```python
from build123d import *

# Parameters (mm, degrees)
SK_MAIN_EXTRUSION_R  = 3.4
MAIN_EXTRUSION_DEPTH = 25


with BuildPart() as part:
    # Sk Main Extrusion → Main Extrusion (new body)
    with BuildSketch(Plane.XY):
        with BuildLine():
            Line((-16.671180212, -4.190076845), (-19.506515107, -5.222054351))
            ThreePointArc((-19.506515107, -5.222054351), (-19.864364033, -5.496641489), (-20, -5.926823816))
            Line((-20, -5.926823816), (-20, -18.5))
            ThreePointArc((-20, -18.5), (-19.560660172, -19.560660172), (-18.5, -20))
            Line((-18.5, -20), (37.5, -20))
            ThreePointArc((37.5, -20), (38.560660172, -19.560660172), (39, -18.5))
            Line((39, -18.5), (39, -16.5))
            ThreePointArc((39, -16.5), (38.560660172, -15.439339828), (37.5, -15))
            Line((37.5, -15), (31.319331136, -15))
            ThreePointArc((31.319331136, -15), (31.252521542, -15.009092387), (31.190571617, -15.035708175))
            Line((31.190571617, -15.035708175), (30.378759519, -15.523494095))
            ThreePointArc((30.378759519, -15.523494095), (30.25, -15.55920227), (30.121240481, -15.523494095))
            Line((30.121240481, -15.523494095), (29.309428383, -15.035708175))
            ThreePointArc((29.309428383, -15.035708175), (29.247478458, -15.009092387), (29.180668864, -15))
            Line((29.180668864, -15), (21, -15))
            ThreePointArc((21, -15), (20.292893219, -14.707106781), (20, -14))
            Line((20, -14), (20, -5.926823816))
            ThreePointArc((20, -5.926823816), (19.864364033, -5.496641489), (19.506515107, -5.222054351))
            Line((19.506515107, -5.222054351), (16.671180212, -4.190076845))
            ThreePointArc((16.671180212, -4.190076845), (16.563886241, -4.175951325), (16.460675177, -4.208493649))
            Line((16.460675177, -4.208493649), (15.111296024, -4.987558066))
            Line((15.111296024, -4.987558066), (14.845251581, -5.718509166))
            Line((14.845251581, -5.718509166), (15.81984631, -8.396186179))
            ThreePointArc((15.81984631, -8.396186179), (15.786489799, -8.811074612), (15.450654467, -9.056960151))
            ThreePointArc((15.450654467, -9.056960151), (12.665882372, -8.933433013), (10.272684887, -7.504160339))
            Line((10.272684887, -7.504160339), (9.309262274, -6.540737726))
            ThreePointArc((9.309262274, -6.540737726), (6.6, 0), (9.309262274, 6.540737726))
            Line((9.309262274, 6.540737726), (10.272684887, 7.504160339))
            ThreePointArc((10.272684887, 7.504160339), (12.665882372, 8.933433013), (15.450654467, 9.056960151))
            ThreePointArc((15.450654467, 9.056960151), (15.786489799, 8.811074612), (15.81984631, 8.396186179))
            Line((15.81984631, 8.396186179), (14.845251581, 5.718509166))
            Line((14.845251581, 5.718509166), (15.111296024, 4.987558066))
            Line((15.111296024, 4.987558066), (16.460675177, 4.208493649))
            ThreePointArc((16.460675177, 4.208493649), (16.563886241, 4.175951325), (16.671180212, 4.190076845))
            Line((16.671180212, 4.190076845), (19.506515107, 5.222054351))
            ThreePointArc((19.506515107, 5.222054351), (19.864364033, 5.496641489), (20, 5.926823816))
            Line((20, 5.926823816), (20, 18.5))
            ThreePointArc((20, 18.5), (19.560660172, 19.560660172), (18.5, 20))
            Line((18.5, 20), (5.926823816, 20))
            ThreePointArc((5.926823816, 20), (5.496641489, 19.864364033), (5.222054351, 19.506515107))
            Line((5.222054351, 19.506515107), (4.190076845, 16.671180212))
            ThreePointArc((4.190076845, 16.671180212), (4.175951325, 16.563886241), (4.208493649, 16.460675177))
            Line((4.208493649, 16.460675177), (4.987558066, 15.111296024))
            Line((4.987558066, 15.111296024), (5.718509166, 14.845251581))
            Line((5.718509166, 14.845251581), (8.396186179, 15.81984631))
            ThreePointArc((8.396186179, 15.81984631), (8.811074612, 15.786489799), (9.056960151, 15.450654467))
            ThreePointArc((9.056960151, 15.450654467), (8.933433013, 12.665882372), (7.504160339, 10.272684887))
            Line((7.504160339, 10.272684887), (6.540737726, 9.309262274))
            ThreePointArc((6.540737726, 9.309262274), (0, 6.6), (-6.540737726, 9.309262274))
            Line((-6.540737726, 9.309262274), (-7.504160339, 10.272684887))
            ThreePointArc((-7.504160339, 10.272684887), (-8.933433013, 12.665882372), (-9.056960151, 15.450654467))
            ThreePointArc((-9.056960151, 15.450654467), (-8.811074612, 15.786489799), (-8.396186179, 15.81984631))
            Line((-8.396186179, 15.81984631), (-5.718509166, 14.845251581))
            Line((-5.718509166, 14.845251581), (-4.987558066, 15.111296024))
            Line((-4.987558066, 15.111296024), (-4.208493649, 16.460675177))
            ThreePointArc((-4.208493649, 16.460675177), (-4.175951325, 16.563886241), (-4.190076845, 16.671180212))
            Line((-4.190076845, 16.671180212), (-5.222054351, 19.506515107))
            ThreePointArc((-5.222054351, 19.506515107), (-5.496641489, 19.864364033), (-5.926823816, 20))
            Line((-5.926823816, 20), (-18.5, 20))
            ThreePointArc((-18.5, 20), (-19.560660172, 19.560660172), (-20, 18.5))
            Line((-20, 18.5), (-20, 5.926823816))
            ThreePointArc((-20, 5.926823816), (-19.864364033, 5.496641489), (-19.506515107, 5.222054351))
            Line((-19.506515107, 5.222054351), (-16.671180212, 4.190076845))
            ThreePointArc((-16.671180212, 4.190076845), (-16.563886241, 4.175951325), (-16.460675177, 4.208493649))
            Line((-16.460675177, 4.208493649), (-15.111296024, 4.987558066))
            Line((-15.111296024, 4.987558066), (-14.845251581, 5.718509166))
            Line((-14.845251581, 5.718509166), (-15.81984631, 8.396186179))
            ThreePointArc((-15.81984631, 8.396186179), (-15.786489799, 8.811074612), (-15.450654467, 9.056960151))
            ThreePointArc((-15.450654467, 9.056960151), (-12.665882372, 8.933433013), (-10.272684887, 7.504160339))
            Line((-10.272684887, 7.504160339), (-9.309262274, 6.540737726))
            ThreePointArc((-9.309262274, 6.540737726), (-6.6, 0), (-9.309262274, -6.540737726))
            Line((-9.309262274, -6.540737726), (-10.272684887, -7.504160339))
            ThreePointArc((-10.272684887, -7.504160339), (-12.665882372, -8.933433013), (-15.450654467, -9.056960151))
            ThreePointArc((-15.450654467, -9.056960151), (-15.786489799, -8.811074612), (-15.81984631, -8.396186179))
            Line((-15.81984631, -8.396186179), (-14.845251581, -5.718509166))
            Line((-14.845251581, -5.718509166), (-15.111296024, -4.987558066))
            Line((-15.111296024, -4.987558066), (-16.460675177, -4.208493649))
            ThreePointArc((-16.460675177, -4.208493649), (-16.563886241, -4.175951325), (-16.671180212, -4.190076845))
        make_face()
        with Locations((14.5, 14.5)):
            Circle(SK_MAIN_EXTRUSION_R, mode=Mode.SUBTRACT)
        Circle(SK_MAIN_EXTRUSION_R, mode=Mode.SUBTRACT)
        with Locations((-14.5, 14.5)):
            Circle(SK_MAIN_EXTRUSION_R, mode=Mode.SUBTRACT)
        with BuildLine():
            Line((-7.441495321, -8.308504679), (-8.577273231, -9.444282589))
            ThreePointArc((-8.577273231, -9.444282589), (-12.430514315, -11.611987193), (-16.849169473, -11.464011904))
            ThreePointArc((-16.849169473, -11.464011904), (-17.295452819, -11.537349181), (-17.5, -11.940719521))
            Line((-17.5, -11.940719521), (-17.5, -17))
            ThreePointArc((-17.5, -17), (-17.353553391, -17.353553391), (-17, -17.5))
            Line((-17, -17.5), (-1.75, -17.5))
            ThreePointArc((-1.75, -17.5), (-1.396446609, -17.353553391), (-1.25, -17))
            Line((-1.25, -17), (-1.25, -6.156094541))
            ThreePointArc((-1.25, -6.156094541), (-1.351026708, -5.854730455), (-1.61328125, -5.675149655))
            ThreePointArc((-1.61328125, -5.675149655), (-2.10305366, -5.51245547), (-2.576734694, -5.307583096))
            ThreePointArc((-2.576734694, -5.307583096), (-4.359333373, -5.153883821), (-5.788120301, -6.230846881))
            ThreePointArc((-5.788120301, -6.230846881), (-6.555931161, -7.316529108), (-7.441495321, -8.308504679))
        make_face(mode=Mode.SUBTRACT)
        with BuildLine():
            Line((1.25, -6.156094541), (1.25, -17))
            ThreePointArc((1.25, -17), (1.396446609, -17.353553391), (1.75, -17.5))
            Line((1.75, -17.5), (17, -17.5))
            ThreePointArc((17, -17.5), (17.353553391, -17.353553391), (17.5, -17))
            Line((17.5, -17), (17.5, -11.940719521))
            ThreePointArc((17.5, -11.940719521), (17.295452819, -11.537349181), (16.849169473, -11.464011904))
            ThreePointArc((16.849169473, -11.464011904), (12.430514315, -11.611987193), (8.577273231, -9.444282589))
            Line((8.577273231, -9.444282589), (7.441495321, -8.308504679))
            ThreePointArc((7.441495321, -8.308504679), (6.555931161, -7.316529108), (5.788120301, -6.230846881))
            ThreePointArc((5.788120301, -6.230846881), (4.359333373, -5.153883821), (2.576734694, -5.307583096))
            ThreePointArc((2.576734694, -5.307583096), (2.10305366, -5.51245547), (1.61328125, -5.675149655))
            ThreePointArc((1.61328125, -5.675149655), (1.351026708, -5.854730455), (1.25, -6.156094541))
        make_face(mode=Mode.SUBTRACT)
    extrude(amount=-MAIN_EXTRUSION_DEPTH)


solid = part.part
```
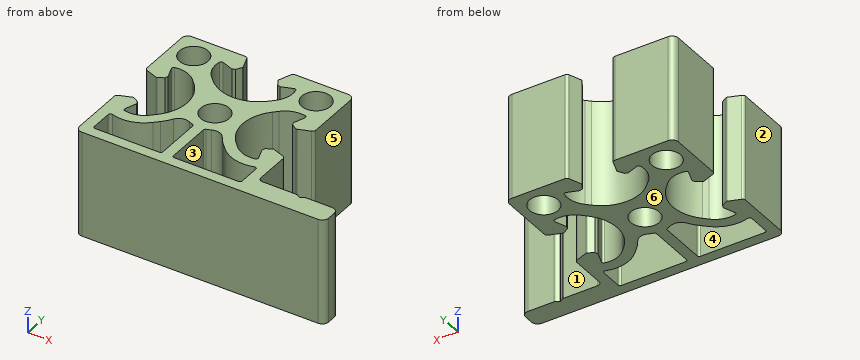
Source: CAD feature listing. Evaluate the final solid. Frame: model axes, mm. Face numbers are marked on the shaded views. A direction names the side the tool comes from. Give positions to 0.01 mm unless a question says otherwise; leave off trailing zeros. Loops run counter-clockwise (first coordinate to the right, second up) from the corner with the lowest first, then second, coordinate; pieces in that order, holes last. Notation, with made-up numbers: (-1.75, -2) -> (4.25, -2) arc R33 cw to (4.25, 37) -> close; hole circle Ø3 at (60.5, 87.25). An arc over 180 degrees is marked (long way). Use a Markdown table: item, result. Add a question column.
(1) Access query for the marked faces 4, 5 and 6. Directions: +Z, -Z, +X, -X, +Y, -Y. A direction counts if a zero-diameter tool reaches every point of the face in a straight line with its end or side. Return the directions, or none.
(2) Section query D-D (y = 13). Output: boundary loops of the cut face in (x, z), then the cut area to 3 significant figures.
(3) Ray query, line 1 (X direction, y = -13.5, z = -16.5); line 2 (Y direction, x = 0, z = -13.25); line 3 (Y direction, x = 12, z = -9). Return the intervals inside material, ascending.
(4) Section query C-C (x = 14). Output: boundary loops of the cut face in (y, z), then the cut area to 3 significant figures.
(5) First-contact query: pin 1 Ø6.5 at (x, z) = (25.5, -11.5) entering from +Y; pin 2 Ø2.5 at (y, z) = (-14.5, -18.5) entering from +X; pin 3 Ø1 at (y, z) = (-3.5, -3.5) entering from +X. Flat tips, straight axial feed; report the tip coordinate or a pass-through.
(6) Section query A-A (x = 0). Output: boundary loops of the cut face in (y, z).
(7) Section query B-B (y = 0). Output: boundary loops of the cut face in (x, z).
(8) Pull-direction query (Y, two-part tool) for the marked faces 1, 2 and 3; classes: +Y half, -Y half, draft (parallel to the pull), parting line (faces both ways), or undercut.
Checked values:
| question | item | result |
|---|---|---|
| 1 | face 4 | +Z, -Z |
| 1 | face 5 | +Z, -Z, +X, +Y |
| 1 | face 6 | -Z, +X, -X, +Y, -Y |
| 2 | outline | (-20, -25) -> (-17.55, -25) -> (-17.55, 0) -> (-20, 0) -> close; (-11.45, -25) -> (-9.02, -25) -> (-9.02, 0) -> (-11.45, 0) -> close; (9.02, -25) -> (11.45, -25) -> (11.45, 0) -> (9.02, 0) -> close; (17.55, -25) -> (20, -25) -> (20, 0) -> (17.55, 0) -> close |
| 2 | area | 244 mm^2 |
| 3 | line 1 | -20 to -17.5, -1.25 to 1.25, 17.5 to 20 |
| 3 | line 2 | -20 to -3.4, 3.4 to 6.6 |
| 3 | line 3 | -20 to -17.5, -11.49 to -8.69, 8.69 to 12.2, 16.8 to 20 |
| 4 | outline | (-20, -25) -> (-17.5, -25) -> (-17.5, 0) -> (-20, 0) -> close; (-11.84, -25) -> (-9.17, -25) -> (-9.17, 0) -> (-11.84, 0) -> close; (9.17, -25) -> (11.14, -25) -> (11.14, 0) -> (9.17, 0) -> close; (17.86, -25) -> (20, -25) -> (20, 0) -> (17.86, 0) -> close |
| 4 | area | 232 mm^2 |
| 5 | pin 1 | y = -15 |
| 5 | pin 2 | x = 38.8 |
| 5 | pin 3 | x = 7.51 |
| 6 | outline | (-20, -25) -> (-3.4, -25) -> (-3.4, 0) -> (-20, 0) -> close; (3.4, -25) -> (6.6, -25) -> (6.6, 0) -> (3.4, 0) -> close |
| 7 | outline | (-6.6, -25) -> (-3.4, -25) -> (-3.4, 0) -> (-6.6, 0) -> close; (3.4, -25) -> (6.6, -25) -> (6.6, 0) -> (3.4, 0) -> close |
| 8 | face 1 | +Y half |
| 8 | face 2 | draft |
| 8 | face 3 | undercut |
